Geometry check sheet. Reference: the model listing, model coordinates, mm. Round coordinates to 2 decimals unless told otherwise and drop trailing zeros. Loops run counter-clockwise (first coordinate to the right, second up) from the corner with the lowest first, then second, coordinate; pieces in that order, holes last. Notation, with made-up numbers: M -15.75,7.25 L 26.25,7.25 A33 ccw 26.25,40.25 Z; hole C 34.5,70.25 d10. An arc over 180 degrees is marked long. Write item = value, one per line.
from build123d import *

# Parameters (mm, degrees)
BOSS_EXTRUDE1_DEPTH       = 1
BOSS_EXTRUDE2_DEPTH       = 5.2
CUTOUT_W                  = 25
CUTOUT_H                  = 60
CUT_EXTRUDE1_DEPTH        = 204.386455918
F_3_0MM_DOWEL_HOLE2_D     = 3.2
F_3_0MM_DOWEL_HOLE2_DEPTH = 1.2
FILLET1_START             = -1
FILLET1_DEPTH             = 7
FILLET2_START             = -1
FILLET2_DEPTH             = 7


with BuildPart() as part:
    # outline → Boss-Extrude1 (new body)
    with BuildSketch(Plane(origin=(0, 0, 0), x_dir=(1, 0, 0), z_dir=(0, 1, 0))):
        Polygon((160.788080985, 105.9953847), (121.597788595, 112.217917805), (22.752080985, 112.217917805), (22.752080985, 32.585832501), (25.688129691, 26.292829341), (39.910245267, 1.671913524), (75.213887712, 15.680109343), (93.764616437, 15.680109343), (112.21601573, 10.581860359), (131.186066133, 10.581860359), (140.397681326, 25.454275085), (160.788080985, 27.045655036), align=None)
        Polygon((121.503115121, 111.017917805), (23.952080985, 111.017917805), (23.952080985, 32.851995342), (26.753439113, 26.847682296), (40.43096447, 3.169545341), (74.984511229, 16.880109343), (93.927351675, 16.880109343), (112.378750968, 11.781860359), (130.517785359, 11.781860359), (139.697830253, 26.603303939), (159.588080985, 28.155649493), (159.588080985, 104.970885583), align=None, mode=Mode.SUBTRACT)
    extrude(amount=BOSS_EXTRUDE1_DEPTH)

    # outline<9> → Boss-Extrude2 (add)
    with BuildSketch(Plane(origin=(0, 0, 0), x_dir=(1, 0, 0), z_dir=(0, 1, 0))):
        Polygon((165.988080985, 110.434880876), (122.008040315, 117.417917805), (17.552080985, 117.417917805), (17.552080985, 31.432460189), (21.071788866, 23.888466533), (37.653795388, -4.817824349), (76.207852469, 10.480109343), (93.059430407, 10.480109343), (111.510829699, 5.381860359), (134.081949487, 5.381860359), (143.430369308, 20.475150048), (165.988080985, 22.235679058), align=None)
        Polygon((121.597788595, 112.217917805), (22.752080985, 112.217917805), (22.752080985, 32.585832501), (25.688129691, 26.292829341), (39.910245267, 1.671913524), (75.213887712, 15.680109343), (93.764616437, 15.680109343), (112.21601573, 10.581860359), (131.186066133, 10.581860359), (140.397681326, 25.454275085), (160.788080985, 27.045655036), (160.788080985, 105.9953847), align=None, mode=Mode.SUBTRACT)
    extrude(amount=BOSS_EXTRUDE2_DEPTH)

    # cutout → Cut-Extrude1 (cut, through all)
    with BuildSketch(Plane(origin=(0, 0, 0), x_dir=(1, 0, 0), z_dir=(0, 1, 0))):
        with Locations((35.252080985, 82.217917805)):
            Rectangle(CUTOUT_W, CUTOUT_H)
        Polygon((17.552080985, 117.417917805), (17.552080985, 52.217917805), (22.752080985, 52.217917805), (22.752080985, 112.217917805), (47.752080985, 112.217917805), (47.752080985, 117.417917805), align=None)
    extrude(amount=CUT_EXTRUDE1_DEPTH, mode=Mode.SUBTRACT)

    # Ø3.0mm Dowel Hole2
    with Locations(Plane.XZ):
        with Locations((84.67493479, -114.817917805), (20.152080985, -32.009146345), (38.782020327, 1.572955412), (75.710870091, -13.080109343), (111.863422715, -7.981860359), (163.388080985, -24.640667047), (163.388080985, -108.215132788), (121.802914455, -114.817917805)):
            Hole(F_3_0MM_DOWEL_HOLE2_D / 2, depth=F_3_0MM_DOWEL_HOLE2_DEPTH)

    # Fillet1: read off the stored shape, not the designer's step
    # Fillet1 outline → Fillet1 (cut)
    with BuildSketch(Plane(origin=(0, 0, 0), x_dir=(1, 0, 0), z_dir=(0, 1, 0)).offset(FILLET1_START)):
        with BuildLine():
            Line((47.752080985, 117.417917805), (47.752080985, 111.017917805))
            ThreePointArc((47.752080985, 111.017917805), (51.424749768, 115.664129056), (57.081604017, 117.417917805))
            Line((57.081604017, 117.417917805), (47.752080985, 117.417917805))
        make_face()
    extrude(amount=FILLET1_DEPTH, mode=Mode.SUBTRACT)

    # Fillet2: read off the stored shape, not the designer's step
    # Fillet2 outline → Fillet2 (cut)
    with BuildSketch(Plane(origin=(0, 0, 0), x_dir=(1, 0, 0), z_dir=(0, 1, 0)).offset(FILLET2_START)):
        with BuildLine():
            Line((17.552080985, 52.217917805), (17.552080985, 42.888394773))
            ThreePointArc((17.552080985, 42.888394773), (19.305869734, 48.545249023), (23.952080985, 52.217917805))
            Line((23.952080985, 52.217917805), (17.552080985, 52.217917805))
        make_face()
    extrude(amount=FILLET2_DEPTH, mode=Mode.SUBTRACT)


solid = part.part
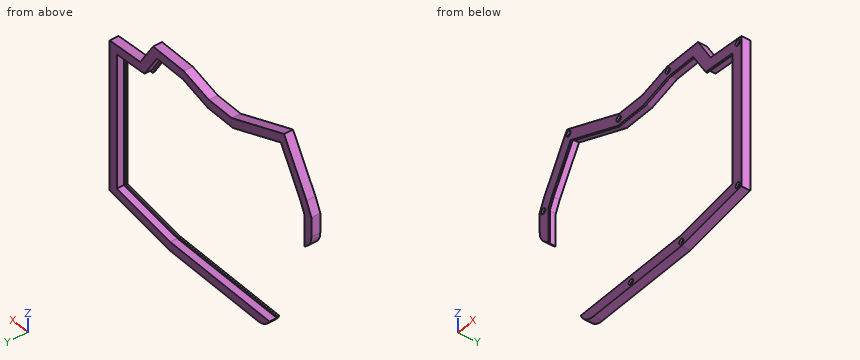
(1) Sectioned sample at C-C on z = -72. Record the cut outline in (x, y), then the cut area to 3 significant figures.
Result set:
outline = M 159.59,0 L 165.99,0 L 165.99,5.2 L 160.79,5.2 L 160.79,1 L 159.59,1 Z
area = 28.2 mm2
(2) Sectioned sample at A-A on x = 150. Record the cut outline in (y, z).
Result set:
outline = M 0,-112.97 L 5.2,-112.97 L 5.2,-107.71 L 1,-107.71 L 1,-106.49 L 0,-106.49 Z; M 0,-27.41 L 1,-27.41 L 1,-26.2 L 5.2,-26.2 L 5.2,-20.99 L 0,-20.99 Z
(3) Depth check by flat-ended pin: pin 1 Ø3.5 at (x, z) = (163.39, -108.22) entering from -Y; pin 2 Ø1.6 at (x, z) = (122, -115.5) entering from -Y; pin 3 Ø1.5 at (x, y) = (118, 4) entering from +Z. Enter the tip coordinate at first touch or a pass-through.
Result set:
pin_1 = 0
pin_2 = 1.2
pin_3 = -5.38
(4) Sectioned sample at B-B on y = 2.55. Record the cut outline in (x, z).
Result set:
outline = M 17.55,-42.89 A10 ccw 22.75,-51.66 L 22.75,-32.59 L 25.69,-26.29 L 39.91,-1.67 L 75.21,-15.68 L 93.76,-15.68 L 112.22,-10.58 L 131.19,-10.58 L 140.4,-25.45 L 160.79,-27.05 L 160.79,-106 L 121.6,-112.22 L 48.31,-112.22 A10 ccw 57.08,-117.42 L 122.01,-117.42 L 165.99,-110.43 L 165.99,-22.24 L 143.43,-20.48 L 134.08,-5.38 L 111.51,-5.38 L 93.06,-10.48 L 76.21,-10.48 L 37.65,4.82 L 21.07,-23.89 L 17.55,-31.43 Z
(5) Sectioned sample at D-D on x = 63.5. Record the cut outline in (y, z), then the cut area to 3 significant figures.
Result set:
outline = M 0,-117.42 L 5.2,-117.42 L 5.2,-112.22 L 1,-112.22 L 1,-111.02 L 0,-111.02 Z; M 0,-12.32 L 1,-12.32 L 1,-11.03 L 5.2,-11.03 L 5.2,-5.44 L 0,-5.44 Z
area = 58.6 mm2
(6) Material ranges on line 1 along Z through (x, y) = (119.5, 2.3); line 2 along Z through (x, y) = (119.5, 0.5); line 3 along X through (y, z) = (1.05, -43), recorded low to high. Write a range as from..to.
Result set:
line_1 = -117.42..-112.22, -10.58..-5.38
line_2 = -117.42..-111.02, -11.78..-5.38
line_3 = 17.55..22.75, 160.79..165.99
